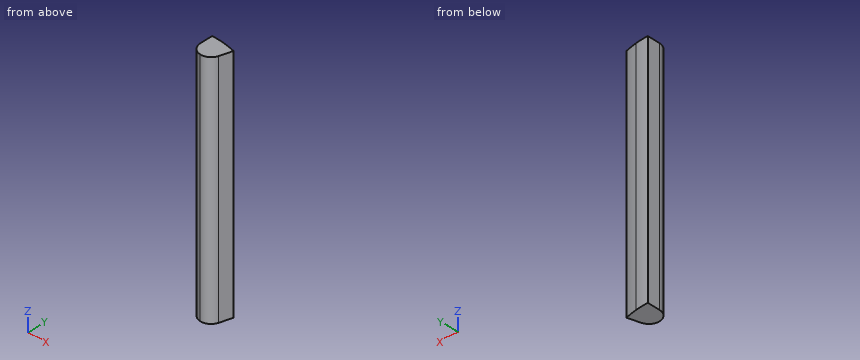
```python
from build123d import *

# Parameters (mm, degrees)
BOSS_EXTRUDE1_DEPTH = 100


with BuildPart() as part:
    # Sketch1 → Boss-Extrude1 (new body)
    with BuildSketch(Plane.XY):
        with BuildLine():
            ThreePointArc((5.152623222, 36.662819266), (1.555688273, 35.597358594), (0, 32.183712234))
            ThreePointArc((0, 32.183712234), (1.109479422, 29.216274726), (3.89362834, 27.704605202))
            Line((3.89362834, 27.704605202), (5.152623222, 36.662819266))
        make_face()
        with BuildLine():
            ThreePointArc((3.89362834, 27.704605202), (6.986596787, 28.390299861), (8.871033436, 30.936970137))
            ThreePointArc((8.871033436, 30.936970137), (9.002232837, 31.554214965), (9.046251562, 32.183712234))
            ThreePointArc((9.046251562, 32.183712234), (7.936772141, 35.151149742), (5.152623222, 36.662819266))
            Line((5.152623222, 36.662819266), (3.89362834, 27.704605202))
        make_face()
        with BuildLine():
            ThreePointArc((9.046251562, 32.183712234), (9.002232837, 31.554214965), (8.871033436, 30.936970137))
            Line((8.871033436, 30.936970137), (10.336400843, 36.047313598))
            ThreePointArc((10.336400843, 36.047313598), (7.796688406, 36.680535028), (5.218991286, 37.135052578))
            Line((5.218991286, 37.135052578), (5.152623222, 36.662819266))
            ThreePointArc((5.152623222, 36.662819266), (7.936772141, 35.151149742), (9.046251562, 32.183712234))
        make_face()
        with BuildLine():
            Line((0, 37.5), (0, 32.183712234))
            ThreePointArc((0, 32.183712234), (1.555688273, 35.597358594), (5.152623222, 36.662819266))
            Line((5.152623222, 36.662819266), (5.218991286, 37.135052578))
            ThreePointArc((5.218991286, 37.135052578), (2.615867765, 37.408651885), (0, 37.5))
        make_face()
    extrude(amount=BOSS_EXTRUDE1_DEPTH)


solid = part.part
```
Could you check a few things on this model? Use its own coordinates, in mm. Round coordinates to 2 decimals unless told otherwise and drop trailing zeros. Loops run counter-clockwise (first coordinate to the right, second up) from the corner with the lowest first, then second, coordinate; pieces in that order, holes last. Notation, with made-up numbers: (-24.5, 32) - (15.5, 32) arc R21 ccw to (15.5, 68) - close; hole circle Ø6 at (-16, 73). An arc over 180 degrees is marked (long way). Answer in a Markdown table with one row per item. Add a question column.
(1) If we section it at A-A (z = 77): Please give me the cut outline in (x, y), plus the area to 3 significant figures.
(2) I'm going to push flat-ended pins straight in: pin 1 (3 mm diameter, centred on x = 2, z = 22, fed in from -Y); pin 2 (1 mm diameter, centred on x = 7, z = 78.5, fed in from -Y). Where does each tip first touch, or does it pass through?
(3) If we section it at C-C (x = 2.5): Please give me the cut outline in (y, z).
(4) If we section it at B-B (y = 33): Please give me the cut outline in (x, z), plus the area to 3 significant figures.
(5) I need wall thicknesses on line 1 along Y through (x, z) = (5.25, 48); line 2 along Y through (x, z) = (7.5, 53.5); line 3 along X through (y, z) = (31, 5). Which ranges of each line are inside material? Lowest first, please.
Model answer:
| question | item | result |
|---|---|---|
| 1 | outline | (0, 32.18) arc R4.52 ccw to (8.87, 30.94) - (10.34, 36.05) arc R37.5 ccw to (0, 37.5) - close |
| 1 | area | 80.1 mm² |
| 2 | pin 1 | stops at y = 27.78 |
| 2 | pin 2 | stops at y = 28.12 |
| 3 | outline | (28.14, 0) - (37.42, 0) - (37.42, 100) - (28.14, 100) - close |
| 4 | outline | (0, 0) - (9.46, 0) - (9.46, 100) - (0, 100) - close |
| 4 | area | 946 mm² |
| 5 | line 1 | y = 27.72 to 37.13 |
| 5 | line 2 | y = 28.78 to 36.74 |
| 5 | line 3 | x = 0.16 to 8.89 |
